Build history of the part. All positions in model axes, mm. A direction names the side the tool comes from. Round coordinates to 2 decimals unless told otherwise and drop trailing zeros. Write each loop counter-clockwise with the first axis right and the second up, starting at its lowest first coordinate (ties: lowest second). Pieces come first, ordered by that corner, then holes.
Item 1: Mould opens along Y. For faces 1 (the cylindrical face through (-11.68, 0.6, 1.53)), 2 (the cylindrical face through (-11.15, 2.93, 1.53)), 3 (the cylindrical face through (-11.68, 5.4, 1.53)), 4 (the flat face through (4, 3, 10.8)) say: +Y half, -Y half, draft (parallel to the pull), parting line (faces both ways), or undercut.
Item 2: 3-axis set-ups, long thin cutter, end or side, ignore diameter. For faces 5 (the flat face through (-1.55, 3, 6)), 6 (the flat face through (5.95, 3, 7)), 7 (the flat face through (-7.66, 2.96, 3.1)): which of +Z, -Z, +X, -X, +Y, -Y reach the whole face in a straight line?
Item 3: Drop flat-ended pins along their axis: pin 1 Ø2 at (x, y) = (1, 4) entering from +Z; pin 2 Ø1.2 at (y, z) = (2, 10) entering from -X; pin 3 Ø1.8 at (x, y) = (-4, 3) entering from -Z; pin 4 Ø0.5 at (x, z) = (-3.5, -4) entering from -Y (3 decimals). Give the stop position or say it passes through.
Item 4: Band-saw the part on C-C, the plane z = 9. Write the cut outline in (x, y).
Item 5: Wall check: probe 1 along X at (y, z) = (4.8, 3.5); probe 2 along X at (y, z) = (4.25, -6.5) (3 decimals); probe 3 along Y at (x, z) = (-9.5, 2.4). Give the ranges that are in metal, low to high.
Item 6: Band-saw the part on D-D, the plane z = -2.75. Write the cut outline in (x, y) (3 decimals), then the cut area to 3 significant figures.
Item 7: Band-saw the part on A-A, the plane x = -9.5. Write the cut outline in (y, z).
Item 8: Band-saw the part on B-B, the plane y = 3. Write the cut outline in (x, z).
```python
from build123d import *

# Parameters (mm, degrees)
F1_DEPTH = 6
F2_R     = 2
F3_R     = 1.65
F4_DEPTH = 3.1
F3_W     = 0.45
F3_H     = 0.45
F5_DEPTH = 7.8
F6_R     = 1.65
F7_DEPTH = 3.1


with BuildPart() as f1:
    # F0 (on Front) → F1 (new body)
    with BuildSketch(Plane.XZ):
        Polygon((-12.25, 0), (12.25, 0), (12.25, 3.1), (5.95, 3.1), (5.95, 10.8), (1.55, 10.8), (1.55, 8.4), (1.95, 8.4), (1.95, 8), (1.55, 8), (1.55, 3.1), (-1.55, 3.1), (-1.55, 8), (-1.95, 8), (-1.95, 8.4), (-1.55, 8.4), (-1.55, 10.8), (-4.95, 10.8), (-5.95, 9.8), (-5.95, 3.1), (-12.25, 3.1), align=None)
    extrude(amount=-F1_DEPTH)

    # F2
    f2_edges = [f1.edges().sort_by_distance(p)[0] for p in [
        (-12.25, 0, 1.55),
        (12.25, 0, 1.55),
        (12.25, 6, 1.55),
        (-12.25, 6, 1.55),
    ]]
    fillet(f2_edges, radius=F2_R)

    # F3 (on face) → F4 (cut, through all)
    with BuildSketch(Plane(origin=(0, 0, 0), x_dir=(1, 0, 0), z_dir=(0, 0, -1))):
        with Locations((-9.5, -3)):
            Circle(F3_R)
        with Locations((9.5, -3)):
            Circle(F3_R)
    extrude(amount=-F4_DEPTH, mode=Mode.SUBTRACT)

    # F3 (on face) → F5 (join)
    with BuildSketch(Plane(origin=(0, 0, 0), x_dir=(1, 0, 0), z_dir=(0, 0, -1))):
        with Locations((-3.8, -1.73)):
            Rectangle(F3_W, F3_H)
        with Locations((-3.8, -4.27)):
            Rectangle(F3_W, F3_H)
        with Locations((3.8, -4.27)):
            Rectangle(F3_W, F3_H)
        with Locations((3.8, -1.73)):
            Rectangle(F3_W, F3_H)
    extrude(amount=F5_DEPTH)

    # F6 (on face) → F7 (cut, through all)
    with BuildSketch(Plane.XY.offset(3.1)):
        with BuildLine():
            Line((10.25, 6), (6.45, 6))
            Line((6.45, 6), (6.45, 0))
            Line((6.45, 0), (10.25, 0))
            ThreePointArc((10.25, 0), (11.6642135624, 0.5857864376), (12.25, 2))
            Line((12.25, 2), (12.25, 4))
            ThreePointArc((12.25, 4), (11.6642135624, 5.4142135624), (10.25, 6))
        make_face()
        with Locations((9.5, 3)):
            Circle(F6_R, mode=Mode.SUBTRACT)
    extrude(amount=-F7_DEPTH, mode=Mode.SUBTRACT)


solid = f1.part
```
Results:
1. face 1: -Y half
1. face 2: undercut
1. face 3: +Y half
1. face 4: draft
2. face 5: +Z, +Y, -Y
2. face 6: +Z, +X, +Y, -Y
2. face 7: +Z, -X, +Y, -Y
3. pin 1: stops at z = 10.8
3. pin 2: stops at x = -5.95
3. pin 3: stops at z = 0
3. pin 4: stops at y = 1.505
4. outline: (-5.95, 0) - (-1.55, 0) - (-1.55, 6) - (-5.95, 6) - close; (1.55, 0) - (5.95, 0) - (5.95, 6) - (1.55, 6) - close
5. probe 1: x = -5.95 to -1.55, 1.55 to 5.95
5. probe 2: x = -4.025 to -3.575, 3.575 to 4.025
5. probe 3: y = 0 to 1.35, 4.65 to 6
6. outline: (-4.025, 1.505) - (-3.575, 1.505) - (-3.575, 1.955) - (-4.025, 1.955) - close; (-4.025, 4.045) - (-3.575, 4.045) - (-3.575, 4.495) - (-4.025, 4.495) - close; (3.575, 1.505) - (4.025, 1.505) - (4.025, 1.955) - (3.575, 1.955) - close; (3.575, 4.045) - (4.025, 4.045) - (4.025, 4.495) - (3.575, 4.495) - close
6. area: 0.810 mm2
7. outline: (0, 0) - (1.35, 0) - (1.35, 3.1) - (0, 3.1) - close; (4.65, 0) - (6, 0) - (6, 3.1) - (4.65, 3.1) - close
8. outline: (-12.25, 0) - (-11.15, 0) - (-11.15, 3.1) - (-12.25, 3.1) - close; (-7.85, 0) - (6.45, 0) - (6.45, 3.1) - (5.95, 3.1) - (5.95, 10.8) - (1.55, 10.8) - (1.55, 8.4) - (1.95, 8.4) - (1.95, 8) - (1.55, 8) - (1.55, 3.1) - (-1.55, 3.1) - (-1.55, 8) - (-1.95, 8) - (-1.95, 8.4) - (-1.55, 8.4) - (-1.55, 10.8) - (-4.95, 10.8) - (-5.95, 9.8) - (-5.95, 3.1) - (-7.85, 3.1) - close
